```python
from build123d import *

# Parameters (mm, degrees)
BOSS_EXTRUDE1_DEPTH = 3.175
CAVITY1_DEPTH       = 3.175


# Read off the part's stored shape, not the designer's step: Cavity1
with BuildPart() as part:
    # Sketch1 → Boss-Extrude1 (new body)
    with BuildSketch(Plane.XY):
        with BuildLine():
            Line((0, 80.613250085), (0, 82.380666667))
            Line((0, 82.380666667), (-3.657727907, 82.380666667))
            ThreePointArc((-3.657727907, 82.380666667), (-7.972232828, 80.689802562), (-9.98902389, 76.517689435))
            Line((-9.98902389, 76.517689435), (-11.122254659, 61.785689435))
            ThreePointArc((-11.122254659, 61.785689435), (-9.450094571, 56.984161746), (-4.790958676, 54.948666667))
            Line((-4.790958676, 54.948666667), (0, 54.948666667))
            Line((0, 54.948666667), (0, 56.800750085))
            ThreePointArc((0, 56.800750085), (-2.38125, 59.182000085), (0, 61.563250085))
            Line((0, 61.563250085), (0, 75.850750085))
            ThreePointArc((0, 75.850750085), (-2.38125, 78.232000085), (0, 80.613250085))
        make_face()
        with BuildLine():
            Line((11.122254659, 61.785689435), (9.98902389, 76.517689435))
            ThreePointArc((9.98902389, 76.517689435), (7.972232828, 80.689802562), (3.657727907, 82.380666667))
            Line((3.657727907, 82.380666667), (0, 82.380666667))
            Line((0, 82.380666667), (0, 80.613250085))
            ThreePointArc((0, 80.613250085), (1.683798023, 79.915798107), (2.38125, 78.232000085))
            ThreePointArc((2.38125, 78.232000085), (1.683798023, 76.548202062), (0, 75.850750085))
            Line((0, 75.850750085), (0, 61.563250085))
            ThreePointArc((0, 61.563250085), (1.683798023, 60.865798107), (2.38125, 59.182000085))
            ThreePointArc((2.38125, 59.182000085), (1.683798023, 57.498202062), (0, 56.800750085))
            Line((0, 56.800750085), (0, 54.948666667))
            Line((0, 54.948666667), (4.790958676, 54.948666667))
            ThreePointArc((4.790958676, 54.948666667), (9.450094571, 56.984161746), (11.122254659, 61.785689435))
        make_face()
    extrude(amount=BOSS_EXTRUDE1_DEPTH)

    # Cavity1 outline → Cavity1 (cut)
    with BuildSketch(Plane.XY):
        Polygon((-7.633502667, 65.742530059), (-7.146479899, 72.073826042), (-10.31212789, 72.317337426), (-10.799150658, 65.986041443), align=None)
        Polygon((10.31212789, 72.317337426), (7.146479899, 72.073826042), (7.633502667, 65.742530059), (10.799150658, 65.986041443), align=None)
    extrude(amount=CAVITY1_DEPTH, mode=Mode.SUBTRACT)


solid = part.part
```
Can you work these out from the model? Positions are in its coordinate system, mm. A direction names the side the tool comes from. Coordinates: 2 decimals unless noted, no trailing zeros. Order: outer loops, then holes, each group sorted by start corner. A loop starts at its lowest first (then second) coordinate and runs counter-clockwise, first axis right, second up. Notation, with made-up numbers: (-32, 13) - (22, 13) arc R6 ccw to (22, 19) - close; hole circle Ø7 at (16, -17). An arc over 180 degrees is marked (long way). Answer in a Markdown table with one row per item.
1. For pin 1 (4 mm diameter, centred on x = 3.5, y = 78.5, fed in from -Z), with a flat end and sliding along its axis, tell me the tip position at first contact or that it passes through.
Reply:
| item | result |
|---|---|
| pin 1 | stops at z = 0 |
2. Suppose I cut it at D-D (y = 68.75). Please give me the cut outline in (x, z) (3 decimals), and give its area (3 significant figures).
Reply:
| item | result |
|---|---|
| outline | (-7.402, 0) - (7.402, 0) - (7.402, 3.175) - (-7.402, 3.175) - close |
| area | 47.0 mm^2 |
3. Suppose I cut it at C-C (x = -1.75). Please give me the cut outline in (y, z) (3 decimals), and give its area (3 significant figures).
Reply:
| item | result |
|---|---|
| outline | (54.949, 0) - (57.567, 0) - (57.567, 3.175) - (54.949, 3.175) - close; (60.797, 0) - (76.617, 0) - (76.617, 3.175) - (60.797, 3.175) - close; (79.847, 0) - (82.381, 0) - (82.381, 3.175) - (79.847, 3.175) - close |
| area | 66.6 mm^2 |
4. If we mould it in two halves opening along Y, with no side actions, what happens to faces 4 (the flat face through (0, 54.949, 2)), 5 (the flat face through (-9.238, 65.866, 1.565)), 6 (the flat face through (-10.96, 63.92, 1.57))? For each: pulls with the +Y half, pulls with the -Y half, needs draft (parallel to the pull), parting line crosses it, or undercut.
Reply:
| item | result |
|---|---|
| face 4 | pulls with the -Y half |
| face 5 | undercut |
| face 6 | pulls with the +Y half |
5. Suppose I cut it at B-B (z = 0.35). Please give me the cut outline in (x, y), and give its area (3 significant figures).
Reply:
| item | result |
|---|---|
| outline | (-11.12, 61.79) arc R6.35 ccw to (-4.79, 54.95) - (4.79, 54.95) arc R6.35 ccw to (11.12, 61.79) - (10.8, 65.99) - (7.63, 65.74) - (7.15, 72.07) - (10.31, 72.32) - (9.99, 76.52) arc R6.35 ccw to (3.66, 82.38) - (-3.66, 82.38) arc R6.35 ccw to (-9.99, 76.52) - (-10.31, 72.32) - (-7.15, 72.07) - (-7.63, 65.74) - (-10.8, 65.99) - close; hole circle Ø4.76 at (0, 59.18); hole circle Ø4.76 at (0, 78.23) |
| area | 470 mm^2 |
6. For faces 1 (the flat face through (9.194, 65.863, 1.565)), 2 (the flat face through (-8.707, 72.194, 1.565)), 3 (the flat face through (8.8, 72.2, 1.6)), which set-ups out of +Z, -Z, +X, -X, +Y, -Y let a thin tool reach every point of the face, with its end or its side?
Reply:
| item | result |
|---|---|
| face 1 | +Z, -Z |
| face 2 | +Z, -Z, -X |
| face 3 | +Z, -Z, +X |
7. If I drill on line 1 along Y through (x, z) = (-0.75, 2.3); line 2 along Y through (x, z) = (1, 2.85); line 3 along X through (y, z) = (72, 1.8), over which ranges is the centre line in solid material (lowest first)?
Reply:
| item | result |
|---|---|
| line 1 | y = 54.95 to 56.92, 61.44 to 75.97, 80.49 to 82.38 |
| line 2 | y = 54.95 to 57.02, 61.34 to 76.07, 80.39 to 82.38 |
| line 3 | x = -7.15 to 7.15 |
8. Suppose I cut it at A-A (x = 8.5). Please give me the cut outline in (y, z) (1 decimal).
Reply:
| item | result |
|---|---|
| outline | (56.1, 0) - (65.8, 0) - (65.8, 3.2) - (56.1, 3.2) - close; (72.2, 0) - (80.1, 0) - (80.1, 3.2) - (72.2, 3.2) - close |
